Verification items for the finished model (mm, model axes). Round coordinates to 2 decimals unless told otherwise and drop trailing zeros. Write each loop counter-clockwise with the first axis right and the second up, starting at its lowest first coordinate (ties: lowest second). Pieces come first, ordered by that corner, then holes. Notation, with made-up numbers: M -14,24 L 19,24 A16 ccw 19,50 Z; hole C 17.5,14.25 d3. An arc over 180 degrees is marked long. Write each question's results on one line, items separated by ' | '.
from build123d import *

# Parameters (mm, degrees)
BOSS_EXTRUDE1_DEPTH = 3.175
FILLET1_R           = 7
FILLET2_R           = 5
SKETCH2_R           = 2.38125
CUT_EXTRUDE1_DEPTH  = 58.715514595
LPATTERN1_COUNT     = 3
LPATTERN1_PITCH     = 12.5


with BuildPart() as part:
    # Sketch1 → Boss-Extrude1 (new body)
    with BuildSketch(Plane.XY):
        with BuildLine():
            Line((-11.618950039, 11), (-36, 11))
            Line((-36, 11), (-36, -34))
            ThreePointArc((-36, -34), (-25, -45), (-14, -34))
            Line((-14, -34), (-14, -11))
            Line((-14, -11), (-11.618950039, -11))
            ThreePointArc((-11.618950039, -11), (16, 0), (-11.618950039, 11))
        make_face()
    extrude(amount=BOSS_EXTRUDE1_DEPTH)

    # Fillet1
    fillet1_edges = [part.edges().sort_by_distance(p)[0] for p in [
        (-36, 11, 1.5875),
    ]]
    fillet(fillet1_edges, radius=FILLET1_R)

    # Fillet2
    # the kernel refuses this fillet: 5 mm, written as the material it adds along each edge
    with BuildSketch(Plane(origin=(-14, -11, 0), x_dir=(1, 0, 0), z_dir=(0, 0, 1))) as fillet2_piece_1:
        with BuildLine():
            CenterArc((5, -4.259237102), FILLET2_R, 121.586822832, 58.413177168)
            Line((0, -4.259237102), (-0.1, -4.259237102))
            Line((-0.1, -4.259237102), (-0.1, 0))
            Line((-0.1, 0), (0, 0.1))
            ThreePointArc((0, 0.1), (1.190524981, 0.1), (2.328670961, 0.085184742))
            Line((2.328670961, 0.085184742), (2.381049961, 0))
        make_face()
    extrude(amount=3.175)

    # Sketch2 → Cut-Extrude1 (cut, through all)
    with BuildSketch(Plane.XY.offset(3.175)):
        Circle(SKETCH2_R)
    cut_extrude1 = extrude(amount=-CUT_EXTRUDE1_DEPTH, mode=Mode.SUBTRACT)

    # LPattern1: Cut-Extrude1 ×3
    with Locations(*[(-i * LPATTERN1_PITCH, 0, 0) for i in range(1, LPATTERN1_COUNT)]):
        add(cut_extrude1, mode=Mode.SUBTRACT)


solid = part.part
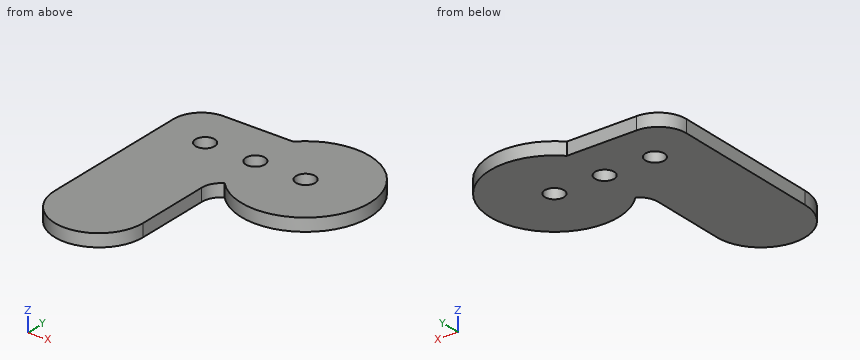
1) Material ranges on line 1 (Y direction, x = 0, z = 1.5); line 2 (Y direction, x = -25, z = 2); line 3 (X direction, y = -1, z = 0.45), recorded low to high. Write a range as [from, to].
Calculated:
line 1: y = [-16, -2.38], [2.38, 16] | line 2: y = [-45, -2.38], [2.38, 11] | line 3: x = [-36, -27.16], [-22.84, -14.66], [-10.34, -2.16], [2.16, 15.97]
2) Depth check by flat-ended pin: P1, Ø1, axis at x = -16, z = 2, coming from the +Y side. Enter the tip coordinate at first touch or a pass-through.
Calculated:
P1: stops at y = 11
3) Sectioned sample at D-D, the plane x = -25. Record the cut outline in (y, z) (3 decimals).
Calculated:
outline: M -45,0 L -2.381,0 L -2.381,3.175 L -45,3.175 Z; M 2.381,0 L 11,0 L 11,3.175 L 2.381,3.175 Z
4) Sectioned sample at A-A, the plane x = 0. Record the cut outline in (y, z) (3 decimals).
Calculated:
outline: M -16,0 L -2.381,0 L -2.381,3.175 L -16,3.175 Z; M 2.381,0 L 16,0 L 16,3.175 L 2.381,3.175 Z
5) Sectioned sample at B-B, the plane z = 2.35. Record the cut outline in (x, y), and give its area (3 significant figures).
Calculated:
outline: M -36,-34 A11 ccw -14,-34 L -14,-15.26 A5 cw -11.62,-11 A16 ccw long -11.62,11 L -29,11 A7 ccw -36,4 Z; hole C -25,0 d4.76; hole C -12.5,0 d4.76; hole C 0,0 d4.76 | area: 1,910 mm²
6) Sectioned sample at C-C, the plane y = 0. Record the cut outline in (x, z) (3 decimals), and give its area (3 significant figures).
Calculated:
outline: M -36,0 L -27.381,0 L -27.381,3.175 L -36,3.175 Z; M -22.619,0 L -14.881,0 L -14.881,3.175 L -22.619,3.175 Z; M -10.119,0 L -2.381,0 L -2.381,3.175 L -10.119,3.175 Z; M 2.381,0 L 16,0 L 16,3.175 L 2.381,3.175 Z | area: 120 mm²
